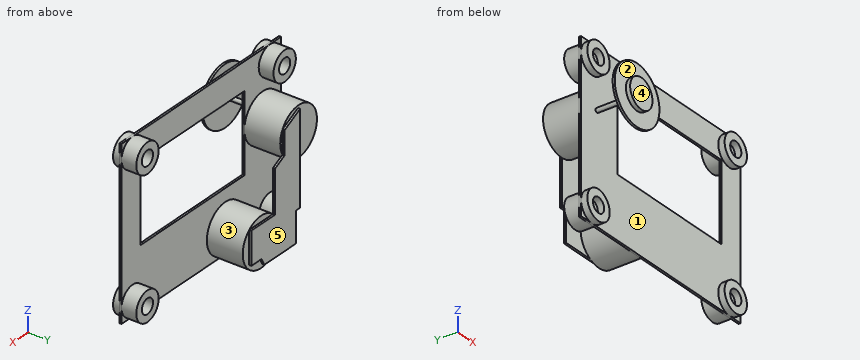
```python
from build123d import *

# Parameters (mm, degrees)
ESQUISSE4_W             = 100
ESQUISSE4_H             = 79
BOSS_EXTRU_3_DEPTH      = 1
BOSS_EXTRU_4_DEPTH      = 7
BOSS_EXTRU_4_DEPTH_BACK = 4
ESQUISSE1_R             = 7
ESQUISSE1_R_2           = 3.5
ESQUISSE6_R             = 11.5
BOSS_EXTRU_5_DEPTH      = 17
BOSS_EXTRU_6_DEPTH      = 1
ESQUISSE8_W             = 65
ESQUISSE8_H             = 37
ENL_V_MAT_EXTRU_1_DEPTH = 1
ESQUISSE9_R             = 1
BOSS_EXTRU_7_DEPTH      = 18
ESQUISSE10_R            = 14
BOSS_EXTRU_8_DEPTH      = 1
ESQUISSE11_R            = 7
BOSS_EXTRU_9_DEPTH      = 2


with BuildPart() as part:
    # Esquisse4 → Boss.-Extru.3 (new body)
    with BuildSketch(Plane(origin=(0, 0, 0), x_dir=(1, 0, 0), z_dir=(0, 1, 0))):
        Rectangle(ESQUISSE4_W, ESQUISSE4_H)
    extrude(amount=-BOSS_EXTRU_3_DEPTH)

    # Esquisse1 → Boss.-Extru.4 (add, two sides: drawn at the far end of the back side and taken through both)
    # profile 1 of 4: a face of its own
    with BuildSketch(Plane(origin=(0, 0, 0), x_dir=(1, 0, 0), z_dir=(0, 1, 0)).offset(-BOSS_EXTRU_4_DEPTH_BACK)):
        with Locations(Location((43, 32.5, 0), (0, 0, 90))):
            Circle(ESQUISSE1_R)
        with Locations(Location((43, 32.5, 0), (0, 0, 90))):
            Circle(ESQUISSE1_R_2, mode=Mode.SUBTRACT)
    # profile 2 of 4: a face of its own
    with BuildSketch(Plane(origin=(0, 0, 0), x_dir=(1, 0, 0), z_dir=(0, 1, 0)).offset(-BOSS_EXTRU_4_DEPTH_BACK)):
        with Locations(Location((-43, 32.5, 0), (0, 0, 90))):
            Circle(ESQUISSE1_R)
        with Locations(Location((-43, 32.5, 0), (0, 0, 90))):
            Circle(ESQUISSE1_R_2, mode=Mode.SUBTRACT)
    # profile 3 of 4: a face of its own
    with BuildSketch(Plane(origin=(0, 0, 0), x_dir=(1, 0, 0), z_dir=(0, 1, 0)).offset(-BOSS_EXTRU_4_DEPTH_BACK)):
        with Locations(Location((-43, -32.5, 0), (0, 0, 270))):
            Circle(ESQUISSE1_R)
        with Locations(Location((-43, -32.5, 0), (0, 0, 90))):
            Circle(ESQUISSE1_R_2, mode=Mode.SUBTRACT)
    # profile 4 of 4: a face of its own
    with BuildSketch(Plane(origin=(0, 0, 0), x_dir=(1, 0, 0), z_dir=(0, 1, 0)).offset(-BOSS_EXTRU_4_DEPTH_BACK)):
        with Locations(Location((43, -32.5, 0), (0, 0, 270))):
            Circle(ESQUISSE1_R)
        with Locations(Location((43, -32.5, 0), (0, 0, 90))):
            Circle(ESQUISSE1_R_2, mode=Mode.SUBTRACT)
    extrude(amount=BOSS_EXTRU_4_DEPTH + BOSS_EXTRU_4_DEPTH_BACK)

    # Esquisse6 → Boss.-Extru.5 (add)
    with BuildSketch(Plane(origin=(0, 0, 0), x_dir=(1, 0, 0), z_dir=(0, 1, 0))):
        with Locations(Location((-38.5, -9.5, 0), (0, 0, 180))):
            Circle(ESQUISSE6_R)
        with Locations(Location((-15, 28, 0), (0, 0, 90))):
            Circle(ESQUISSE6_R)
    extrude(amount=BOSS_EXTRU_5_DEPTH)

    # Esquisse7 → Boss.-Extru.6 (add)
    with BuildSketch(Plane(origin=(0, 17, 0), x_dir=(1, 0, 0), z_dir=(0, 1, 0))):
        Polygon((-38.143774149, -19.88751618), (-28.414215556, -15.025120102), (-28.414215556, -3.974879898), (-22.428299765, -0.98338823), (-22.428299765, 19.221027247), (-7.571700235, 19.221027247), (-7.571700235, 34.680148422), (-13.988712335, 34.680148422), (-15.667356388, 38.039082045), (-35.613243864, 38.039082045), (-35.613243864, 23.559466539), (-38.143774149, 23.559466539), (-38.143774149, 0), align=None)
    extrude(amount=BOSS_EXTRU_6_DEPTH)

    # Esquisse8 → Enlèv. mat.-Extru.1 (cut)
    with BuildSketch(Plane(origin=(0, 0, 0), x_dir=(1, 0, 0), z_dir=(0, 1, 0))):
        with Locations((5.5, -8)):
            Rectangle(ESQUISSE8_W, ESQUISSE8_H)
    extrude(amount=-ENL_V_MAT_EXTRU_1_DEPTH, mode=Mode.SUBTRACT)

    # Esquisse9 → Boss.-Extru.7 (add)
    with BuildSketch(Plane.XZ.offset(1)):
        with Locations(Location((-40, 11.5, 0), (0, 0, 270))):
            Circle(ESQUISSE9_R)
    extrude(amount=BOSS_EXTRU_7_DEPTH)

    # Esquisse10 → Boss.-Extru.8 (add)
    with BuildSketch(Plane.XZ.offset(19)):
        with Locations(Location((-40, 11.5, 0), (0, 0, 270))):
            Circle(ESQUISSE10_R)
    extrude(amount=BOSS_EXTRU_8_DEPTH)

    # Esquisse11 → Boss.-Extru.9 (add)
    with BuildSketch(Plane(origin=(0, -20, 0), x_dir=(-1, 0, 0), z_dir=(0, -1, 0))):
        with Locations(Location((40, -11.5, 0), (0, 0, 90))):
            Circle(ESQUISSE11_R)
    extrude(amount=BOSS_EXTRU_9_DEPTH)


solid = part.part
```
Input: part model. Units: mm. Frame: model coordinates. Face numbers are marked on the shaded views. A direction names the side the tool comes from. Give positions to 0.01 mm unless a question says otherwise; leave off trailing zeros. Order: outer loops, then holes, each group sorted by start corner. A loop starts at its lowest first (then second) coordinate and runs counter-clockwise, first axis right, second up.
1. Section A-A on z = -14.5. Return the cut outline in (x, y).
Derived:
outline: (-50, -1) - (50, -1) - (50, 0) - (-50, 0) - close; (-38.14, 17) - (-22.43, 17) - (-22.43, 18) - (-38.14, 18) - close
2. Pin query (flat end, axial travel): pin 1 (5.5 mm diameter, centred on x = -47.5, z = 37, fed in from -Y); pin 2 (12 mm diameter, centred on x = -14, z = 18, fed in from -Y); pin 3 (4 mm diameter, centred on x = -28, z = 11.5, fed in from -Y); pin 4 (0.8 mm diameter, centred on y = -0.5, z = 9, fed in from -X). Return the tip coordinate at first contact, or that it passes through.
Derived:
pin 1: stops at y = -4
pin 2: passes through
pin 3: stops at y = -20
pin 4: stops at x = -50
3. Section C-C on y = -17. Return the cut outline in (x, z), and give its area (3 significant figures).
Derived:
outline: circle Ø2 at (-40, 11.5)
area: 3.14 mm2
4. Mould query, pull axis Y, two halves, no side actions, for the marked faces 3, 4 and 5. Classes: released by +Y, released by -Y, zero draft, split by the parting line, or undercut.
Derived:
face 3: undercut
face 4: released by -Y
face 5: released by +Y
5. Reachability of the marked faces 1 and 2 from +Z, -Z, +X, -X, +Y, -Y: full face, straight path, thin tool, end or side. Return the list, or none.
Derived:
face 1: none
face 2: -Y
6. Section B-B on y = 10.5. Return the cut outline in (x, z), and give its area (3 significant figures).
Derived:
outline: circle Ø23 at (-38.5, 9.5); circle Ø23 at (-15, -28)
area: 831 mm2
7. Material intervals for L1, parallel to Z at x = -43, y = -2; L2, parallel to X at y = -2.6, z = 32.5; L3, parallel to Z at x = -47.5, y = 2, sorted ascending.
Derived:
L1: z = -39.5 to -36, -29 to -25.5, 25.5 to 29, 36 to 39.5
L2: x = -50 to -46.5, -39.5 to -36, 36 to 39.5, 46.5 to 50
L3: z = -37.86 to -27.14, 2.34 to 16.66, 27.14 to 37.86
